Design review of the part built by this model. Coordinates are the model's own, in mm. Coordinates: 2 decimals unless noted, no trailing zeros. Write each loop counter-clockwise with the first axis right and the second up, starting at its lowest first coordinate (ties: lowest second). Pieces come first, ordered by that corner, then holes. Notation, with made-up numbers: (66, -20.5) - (93, -20.5) arc R20 cw to (93, 2.5) - close; hole circle Ø7 at (45.5, -25). An arc over 180 degrees is marked (long way). Answer as CSV lines item,"result". Start each with the question number.
Q1. Clearance check with flat-ended pins moving along their axes: pin 1 (2.5 mm diameter, centred on x = 140.11, z = -109.64, fed in from +Y); pin 2 (1.8 mm diameter, centred on x = -178, y = 4.5, fed in from -Z); pin 3 (1.8 mm diameter, centred on y = 2.5, z = 148, fed in from -X). State where each tip first meets the part, or that it passes through.
Q2. For line 1 along X through (y, z) = (3.8, 22.44); line 2 along Z through (x, y) = (140.11, 2.6); line 3 along Z through (x, y) = (160, 1.95), list the stretches that pass through material, from the lowest coordinate up. Write a range as [from, to].
Q3. We need section A-A (z = 120). Write out the cut boundary in (x, y).
Q4. We need section B-B (y = 5.1). State how many separate pieces and enclosed holes the cut face has, plus the area to 3 significant figures.
from build123d import *

# Parameters (mm, degrees)
BASE_PLATE_W        = 380
BASE_PLATE_H        = 325
BASE_PLATE_R        = 1.5
BASE_PLATE_R_2      = 2.5
BASE_PLATE_W_2      = 55
BASE_PLATE_H_2      = 25
BOSS_EXTRUDE1_DEPTH = 6
SKETCH1_W           = 20
SKETCH1_H           = 20
CUT_EXTRUDE1_DEPTH  = 10
SKETCH2_R           = 2.55
CUT_EXTRUDE2_DEPTH  = 10


with BuildPart() as part:
    # Base Plate → Boss-Extrude1 (new body)
    with BuildSketch(Plane(origin=(0, 0, 0), x_dir=(1, 0, 0), z_dir=(0, 1, 0))):
        Rectangle(BASE_PLATE_W, BASE_PLATE_H)
        with Locations(Location((-139.29, -94.83, 0), (0, 0, 270))):
            Circle(BASE_PLATE_R, mode=Mode.SUBTRACT)
        with Locations(Location((-14.83, -22.44, 0), (0, 0, 270))):
            Circle(BASE_PLATE_R, mode=Mode.SUBTRACT)
        with Locations(Location((-139.29, -22.44, 0), (0, 0, 270))):
            Circle(BASE_PLATE_R, mode=Mode.SUBTRACT)
        with Locations(Location((-139.29, 132.5, 0), (0, 0, 270))):
            Circle(BASE_PLATE_R, mode=Mode.SUBTRACT)
        with Locations(Location((-14.83, 132.5, 0), (0, 0, 270))):
            Circle(BASE_PLATE_R, mode=Mode.SUBTRACT)
        with Locations(Location((-14.83, -94.83, 0), (0, 0, 270))):
            Circle(BASE_PLATE_R, mode=Mode.SUBTRACT)
        with Locations(Location((140.11, -94.83, 0), (0, 0, 270))):
            Circle(BASE_PLATE_R, mode=Mode.SUBTRACT)
        with Locations(Location((140.11, -22.44, 0), (0, 0, 270))):
            Circle(BASE_PLATE_R, mode=Mode.SUBTRACT)
        with Locations(Location((140.11, 109.64, 0), (0, 0, 270))):
            Circle(BASE_PLATE_R, mode=Mode.SUBTRACT)
        with Locations(Location((-180, -152.5, 0), (0, 0, 270))):
            Circle(BASE_PLATE_R_2, mode=Mode.SUBTRACT)
        with Locations(Location((180, -152.5, 0), (0, 0, 270))):
            Circle(BASE_PLATE_R_2, mode=Mode.SUBTRACT)
        with Locations(Location((-180, 152.5, 0), (0, 0, 270))):
            Circle(BASE_PLATE_R_2, mode=Mode.SUBTRACT)
        with Locations(Location((180, 152.5, 0), (0, 0, 270))):
            Circle(BASE_PLATE_R_2, mode=Mode.SUBTRACT)
        with Locations((41.5, -127.33)):
            Rectangle(BASE_PLATE_W_2, BASE_PLATE_H_2, mode=Mode.SUBTRACT)
        with Locations((-53.5, -127.33)):
            Rectangle(BASE_PLATE_W_2, BASE_PLATE_H_2, mode=Mode.SUBTRACT)
    extrude(amount=BOSS_EXTRUDE1_DEPTH)

    # Sketch1 → Cut-Extrude1 (cut)
    with BuildSketch(Plane(origin=(0, 6, 0), x_dir=(1, 0, 0), z_dir=(0, 1, 0))):
        with Locations((-180, 152.5)):
            Rectangle(SKETCH1_W, SKETCH1_H)
        with Locations((180, 152.5)):
            Rectangle(SKETCH1_W, SKETCH1_H)
        with Locations((180, -152.5)):
            Rectangle(SKETCH1_W, SKETCH1_H)
        with Locations((-180, -152.5)):
            Rectangle(SKETCH1_W, SKETCH1_H)
    extrude(amount=-CUT_EXTRUDE1_DEPTH, mode=Mode.SUBTRACT)

    # Sketch2 → Cut-Extrude2 (cut)
    with BuildSketch(Plane.XZ):
        with Locations(Location((-160, 152.5, 0), (0, 0, 270))):
            Circle(SKETCH2_R)
        with Locations(Location((-180, 132.5, 0), (0, 0, 270))):
            Circle(SKETCH2_R)
        with Locations(Location((-180, -132.5, 0), (0, 0, 270))):
            Circle(SKETCH2_R)
        with Locations(Location((-160, -152.5, 0), (0, 0, 270))):
            Circle(SKETCH2_R)
        with Locations(Location((160, -152.5, 0), (0, 0, 270))):
            Circle(SKETCH2_R)
        with Locations(Location((180, -132.5, 0), (0, 0, 270))):
            Circle(SKETCH2_R)
        with Locations(Location((180, 132.5, 0), (0, 0, 270))):
            Circle(SKETCH2_R)
        with Locations(Location((160, 152.5, 0), (0, 0, 270))):
            Circle(SKETCH2_R)
    extrude(amount=-CUT_EXTRUDE2_DEPTH, mode=Mode.SUBTRACT)


solid = part.part
Results list:
1,pin 1,"passes through"
1,pin 2,"stops at z = -142.5"
1,pin 3,"stops at x = -170"
2,line 1,"x = [-190, -140.79], [-137.79, -16.33], [-13.33, 138.61], [141.61, 190]"
2,line 2,"z = [-162.5, -111.14], [-108.14, 20.94], [23.94, 93.33], [96.33, 162.5]"
2,line 3,"z = [-162.5, -155.05], [-149.95, 149.95], [155.05, 162.5]"
3,outline,"(-190, 0) - (-81, 0) - (-81, 6) - (-190, 6) - close; (-26, 0) - (14, 0) - (14, 6) - (-26, 6) - close; (69, 0) - (190, 0) - (190, 6) - (69, 6) - close"
4,separate pieces,"1"
4,enclosed holes,"19"
4,area,"119,000 mm2"
